from build123d import *

# Parameters (mm, degrees)
F0_W     = 58.8
F0_H     = 58.8
F1_DEPTH = 40
F2_W     = 40.64
F2_H     = 40.64
F3_DEPTH = 40.001
F4_R     = 2.5
F5_DEPTH = 8
F6_R     = 12.7
F7_R     = 5


with BuildPart() as f1:
    # F0 (on Top) → F1 (new body)
    with BuildSketch(Plane.XY):
        Rectangle(F0_W, F0_H)
    extrude(amount=F1_DEPTH)

    # F2 (on face) → F3 (cut, through all)
    with BuildSketch(Plane.XY.offset(40)):
        Rectangle(F2_W, F2_H)
    extrude(amount=-F3_DEPTH, mode=Mode.SUBTRACT)

    # F4 (on face) → F5 (cut)
    with BuildSketch(Plane(origin=(0, 0, 0), x_dir=(1, 0, 0), z_dir=(0, 0, -1))):
        with Locations((-24.86, 0)):
            Circle(F4_R)
        with Locations((0, 24.86)):
            Circle(F4_R)
        with Locations((24.86, 0)):
            Circle(F4_R)
        with Locations((0, -24.86)):
            Circle(F4_R)
    extrude(amount=-F5_DEPTH, mode=Mode.SUBTRACT)

    # F6
    f6_edges = [f1.edges().sort_by_distance(p)[0] for p in [
        (-20.32, 20.32, 20),
        (20.32, 20.32, 20),
        (20.32, -20.32, 20),
        (-20.32, -20.32, 20),
    ]]
    fillet(f6_edges, radius=F6_R)

    # F7
    f7_edges = [f1.edges().sort_by_distance(p)[0] for p in [
        (-29.4, -29.4, 20),
        (-29.4, 29.4, 20),
        (29.4, -29.4, 20),
        (29.4, 29.4, 20),
    ]]
    fillet(f7_edges, radius=F7_R)


solid = f1.part
For this review, take the finished solid that the model builds, in its own axes (mm). A direction names the side the tool comes from. Give positions to 0.01 mm unless a question says otherwise; leave off trailing zeros. Order: outer loops, then holes, each group sorted by start corner. A loop starts at its lowest first (then second) coordinate and runs counter-clockwise, first axis right, second up. Notation, with made-up numbers: M -21.75,53 L 19.25,53 A12 cw 19.25,71 Z; hole C 74,-20.75 d5. An arc over 180 degrees is marked long. Answer in a Markdown table with one row per item. Add a question column.
(1) For faces 1 (the face through (20.32, 0, 20)), 2 (the face through (-25, 0, 8)), 3 (the face through (-29.4, 0, 20)), list the 3-axis set-ups (+Z, -Z, +X, -X, +Y, -Y) from which the entire face can be reached by the end or side of a thin tool; tool diameter is ignored.
(2) Wall thickness on probe 1 along Y at (x, z) = (0, 2.25); probe 2 along X at (y, z) = (-2, 32.5): over which ranges is each line inside the solid? List them lowest first. Write a range as [from, to].
(3) Consider section B-B on x = 0. State the section outline as (y, z) points.
(4) For pin 1 (2.5 mm diameter, centred on x = 24, y = 1, fed in from -Z); pin 2 (1.5 mm diameter, centred on x = -24, y = 0.5, fed in from -Z), all flat-tipped, find the tip position at first contact; note any pin that passes through.
(5) Consider section A-A on y = -5.5. State the section outline as (x, z) points, and give its area (3 significant figures).
(6) Mouldability with a two-part tool opening along Y and no side actions: class faces 4 (the face through (0, -29.4, 20)), 5 (the face through (-0.33, 22.38, 3.94)), 6 (the face through (-20, 13, 40)) as +Y half, -Y half, draft (parallel to the pull), parting line (faces both ways), or undercut.
(7) Consider section D-D on x = 14. State the section outline as (y, z) points.
(8) Consider section C-C on z = 32. State the section outline as (x, y) points, and give its area (3 significant figures).
Evaluation:
| question | item | result |
|---|---|---|
| 1 | face 1 | +Z, -Z |
| 1 | face 2 | -Z |
| 1 | face 3 | +Z, -Z, -X, +Y, -Y |
| 2 | probe 1 | y = [-29.4, -27.36], [-22.36, -20.32], [20.32, 22.36], [27.36, 29.4] |
| 2 | probe 2 | x = [-29.4, -20.32], [20.32, 29.4] |
| 3 | outline | M -29.4,0 L -27.36,0 L -27.36,8 L -22.36,8 L -22.36,0 L -20.32,0 L -20.32,40 L -29.4,40 Z; M 20.32,0 L 22.36,0 L 22.36,8 L 27.36,8 L 27.36,0 L 29.4,0 L 29.4,40 L 20.32,40 Z |
| 4 | pin 1 | stops at z = 0 |
| 4 | pin 2 | stops at z = 8 |
| 5 | outline | M -29.4,0 L -20.32,0 L -20.32,40 L -29.4,40 Z; M 20.32,0 L 29.4,0 L 29.4,40 L 20.32,40 Z |
| 5 | area | 726 mm^2 |
| 6 | face 4 | -Y half |
| 6 | face 5 | undercut |
| 6 | face 6 | draft |
| 7 | outline | M -29.4,0 L -18.6,0 L -18.6,40 L -29.4,40 Z; M 18.6,0 L 29.4,0 L 29.4,40 L 18.6,40 Z |
| 8 | outline | M -29.4,-24.4 A5 ccw -24.4,-29.4 L 24.4,-29.4 A5 ccw 29.4,-24.4 L 29.4,24.4 A5 ccw 24.4,29.4 L -24.4,29.4 A5 ccw -29.4,24.4 Z; hole M -20.32,-7.62 A12.7 ccw -7.62,-20.32 L 7.62,-20.32 A12.7 ccw 20.32,-7.62 L 20.32,7.62 A12.7 ccw 7.62,20.32 L -7.62,20.32 A12.7 ccw -20.32,7.62 Z |
| 8 | area | 1,920 mm^2 |
